from build123d import *

# Parameters (mm, degrees)
SKETCH002_R      = 1.65
SKETCH002_R_2    = 1.25
SKETCH002_R_3    = 7.6
EXTRUDE001_DEPTH = 6
SKETCH003_R      = 11.8
POCKET001_DEPTH  = 2
POCKET002_DEPTH  = 3.5


with BuildPart() as part:
    # Sketch002 → Extrude001 (new body)
    with BuildSketch(Plane(origin=(0, -257.5, 260.94116), x_dir=(-1, 0, 0), z_dir=(0, 0, -1))):
        Polygon((278.411955, 248.765839), (312.411955, 248.765839), (316.411955, 244.765839), (316.411955, 210.765839), (312.411955, 206.765839), (278.411955, 206.765839), (274.411955, 210.765839), (274.411955, 244.765839), align=None)
        with Locations((279.911955, 243.265839)):
            Circle(SKETCH002_R, mode=Mode.SUBTRACT)
        with Locations((310.911955, 243.265839)):
            Circle(SKETCH002_R, mode=Mode.SUBTRACT)
        with Locations((310.911955, 212.265839)):
            Circle(SKETCH002_R, mode=Mode.SUBTRACT)
        with Locations((279.911955, 212.265839)):
            Circle(SKETCH002_R, mode=Mode.SUBTRACT)
        with Locations((295.411955, 237.265839)):
            Circle(SKETCH002_R_2, mode=Mode.SUBTRACT)
        with Locations((303.639196, 223.015839)):
            Circle(SKETCH002_R_2, mode=Mode.SUBTRACT)
        with Locations((287.184713, 223.015839)):
            Circle(SKETCH002_R_2, mode=Mode.SUBTRACT)
        with Locations((295.411955, 227.765839)):
            Circle(SKETCH002_R_3, mode=Mode.SUBTRACT)
    extrude(amount=-EXTRUDE001_DEPTH)


with BuildPart() as part_1:
    # Extrude001 placement: moved
    add(part.part.moved(Location((295.412, 29.7342, -218))))

    # Sketch003 → Pocket001 (cut)
    with BuildSketch(Plane(origin=(295.412, 29.7342, 42.94116), x_dir=(1, 0, 0), z_dir=(0, 0, -1))):
        with Locations((-295.411955, 29.734161)):
            Circle(SKETCH003_R)
    extrude(amount=-POCKET001_DEPTH, mode=Mode.SUBTRACT)

    # Sketch004 → Pocket002 (cut)
    with BuildSketch(Plane(origin=(295.412, 29.7342, 42.94116), x_dir=(1, 0, 0), z_dir=(0, 0, -1))):
        Polygon((-313.811955, 43.559845), (-310.911955, 41.885529), (-308.011955, 43.559845), (-308.011955, 46.908477), (-310.911955, 48.582792), (-313.811955, 46.908477), align=None)
        Polygon((-279.911955, 41.885529), (-277.011955, 43.559845), (-277.011955, 46.908477), (-279.911955, 48.582792), (-282.811955, 46.908477), (-282.811955, 43.559845), align=None)
        Polygon((-279.911955, 17.582792), (-282.811955, 15.908477), (-282.811955, 12.559845), (-279.911955, 10.885529), (-277.011955, 12.559845), (-277.011955, 15.908477), align=None)
        Polygon((-310.911955, 17.582792), (-313.811955, 15.908477), (-313.811955, 12.559845), (-310.911955, 10.885529), (-308.011955, 12.559845), (-308.011955, 15.908477), align=None)
    extrude(amount=-POCKET002_DEPTH, mode=Mode.SUBTRACT)


solid = part_1.part
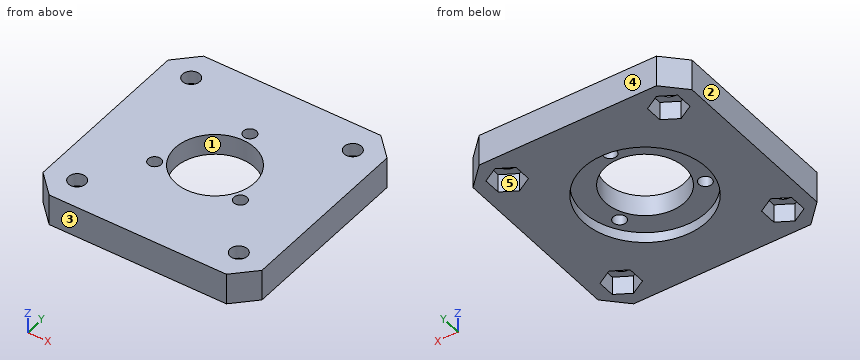
Part model, mm, in its own coordinate system. Face numbers are marked on the shaded views. A direction names the side the tool comes from. Coordinates: 2 decimals unless noted, no trailing zeros. Order: outer loops, then holes, each group sorted by start corner. A loop starts at its lowest first (then second) coordinate and runs counter-clockwise, first axis right, second up. Notation, with made-up numbers: M -9.75,19.25 L 17.25,19.25 A27 ccw 17.25,46.25 Z; hole C -30.75,73 d1. An arc over 180 degrees is marked long. One line per question, with ' | ' between items.
Q1. Slice it at C-C (y = 2.5). Give the cut face in (x, z).
A:
outline: M -21,42.94 L -11.53,42.94 L -11.53,44.94 L -7.18,44.94 L -7.18,48.94 L -21,48.94 Z; M 7.18,44.94 L 11.53,44.94 L 11.53,42.94 L 21,42.94 L 21,48.94 L 7.18,48.94 Z
Q2. Two-plate mould, pull along Y, no slides. Class the marked faces 1, 2 and 3: +Y half, -Y half, draft (parallel to the pull), parting line (faces both ways), or undercut.
A:
face 1: undercut | face 2: draft | face 3: -Y half
Q3. Slice it at B-B (z = 48). Count the separate pieces of the cut face and the enclosed holes in it, and give its area (3 significant figures).
A:
separate pieces: 1 | enclosed holes: 8 | area: 1,500 mm^2
Q4. Pin check, flat tips, straight feed: P1, Ø3, axis at x = 0, y = 9.5, coming from the -Z side; P2, Ø4, axis at x = -15.5, y = -15.5, coming from the -Z side. Stop position of each tip, or through.
A:
P1: stops at z = 44.94 | P2: stops at z = 46.44
Q5. 3-axis set-ups, long thin cutter, end or side, ignore diameter. For the marked faces 4 and 5: which of +Z, -Z, +X, -X, +Y, -Y reach the whole face in a straight line?
A:
face 4: +Z, -Z, +X, -X, +Y | face 5: -Z
Q6. Slice it at D-D (x = 14.5). Give the cut face in (y, z).
A:
outline: M -21,42.94 L -18.27,42.94 L -18.27,46.44 L -16.81,46.44 L -16.81,48.94 L -21,48.94 Z; M -14.19,46.44 L -12.73,46.44 L -12.73,42.94 L 12.73,42.94 L 12.73,46.44 L 14.19,46.44 L 14.19,48.94 L -14.19,48.94 Z; M 16.81,46.44 L 18.27,46.44 L 18.27,42.94 L 21,42.94 L 21,48.94 L 16.81,48.94 Z
Q7. Slice it at A-A (x = -5). Give the cut face in (y, z).
A:
outline: M -21,42.94 L -10.69,42.94 L -10.69,44.94 L -5.72,44.94 L -5.72,48.94 L -21,48.94 Z; M 5.72,44.94 L 10.69,44.94 L 10.69,42.94 L 21,42.94 L 21,48.94 L 5.72,48.94 Z
Q8. Drill centre lines: line 1 (X direction, y = 17, z = 45.5); line 2 (X direction, y = 17, z = 48.75); line 3 (Y direction, x = 17.5, z = 46). Where is each one in solid material? Low to high.
A:
line 1: x = -21 to -18.4, -12.6 to 12.6, 18.4 to 21 | line 2: x = -21 to -16.19, -14.81 to 14.81, 16.19 to 21 | line 3: y = -20.5 to -17.69, -13.31 to 13.31, 17.69 to 20.5
